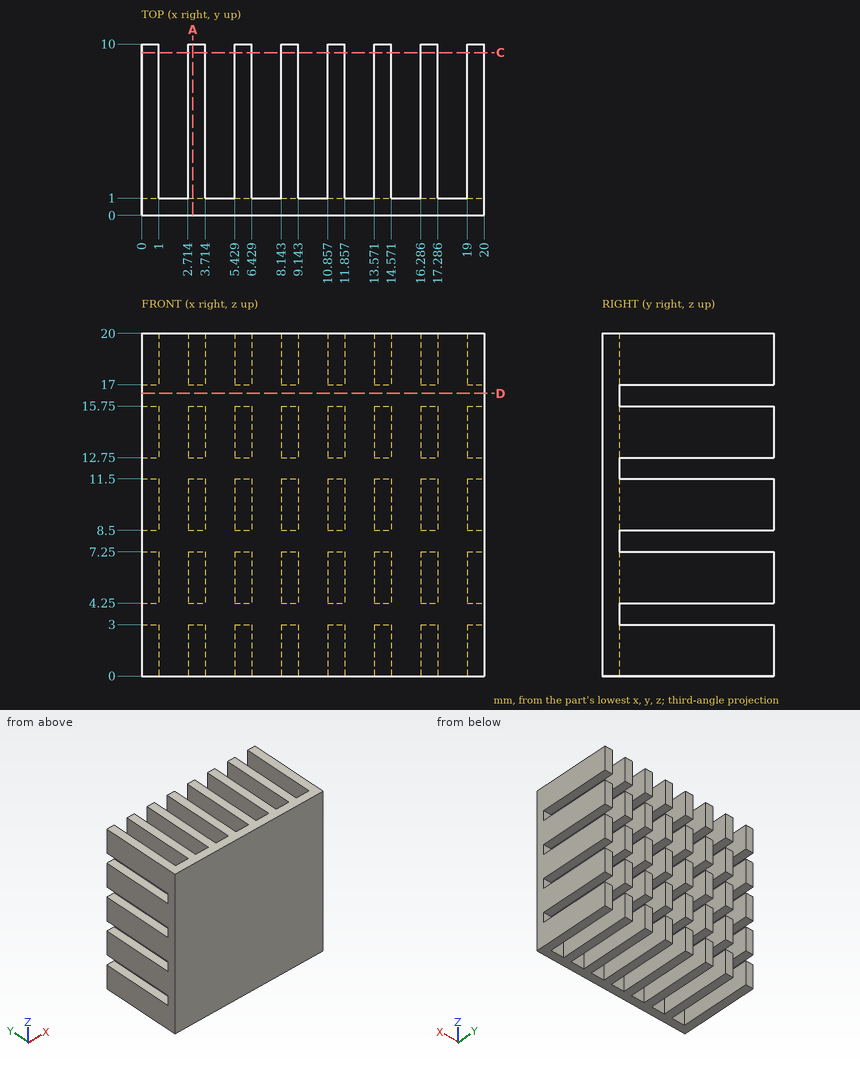
Check sheet for the drawn part. Datum: minimum x, y, z corner. Units: mm. Round coordinates to 2 decimals unless told otherwise and drop trailing zeros. Loops run counter-clockwise (first coordinate to the right, second up) from the corner with the lowest first, then second, coordinate; pieces in that order, holes last. Notation, with made-up numbers: M -33,47 L 25,47 A13 ccw 25,58 Z; hole C -29,46 d4. An arc over 180 degrees is marked long. One line per question, with ' | ' between items. Start each with the question number.
Item 1: Scan lines: probe 1 along Z at (x, y) = (11.25, 4.75); probe 2 along Y at (x, z) = (10.25, 3.5). Record each from-to range of solid material in increasing order.
Item 2: Section check D-D (z = 16.5). Record the boundary of the cut face in (x, y), and give its area (3 significant figures).
Item 3: Section check C-C (y = 9.5). State how many separate pieces and enclosed holes the cut face has, and give its area (3 significant figures).
Item 4: Section check A-A (x = 3). Record the boundary of the cut face in (y, z).
Worked out:
1) probe 1: 0 to 3, 4.25 to 7.25, 8.5 to 11.5, 12.75 to 15.75, 17 to 20 | probe 2: 0 to 1
2) outline: M 0,0 L 20,0 L 20,1 L 0,1 Z | area: 20.0 mm^2
3) separate pieces: 40 | enclosed holes: 0 | area: 120 mm^2
4) outline: M 0,0 L 10,0 L 10,3 L 1,3 L 1,4.25 L 10,4.25 L 10,7.25 L 1,7.25 L 1,8.5 L 10,8.5 L 10,11.5 L 1,11.5 L 1,12.75 L 10,12.75 L 10,15.75 L 1,15.75 L 1,17 L 10,17 L 10,20 L 0,20 Z
